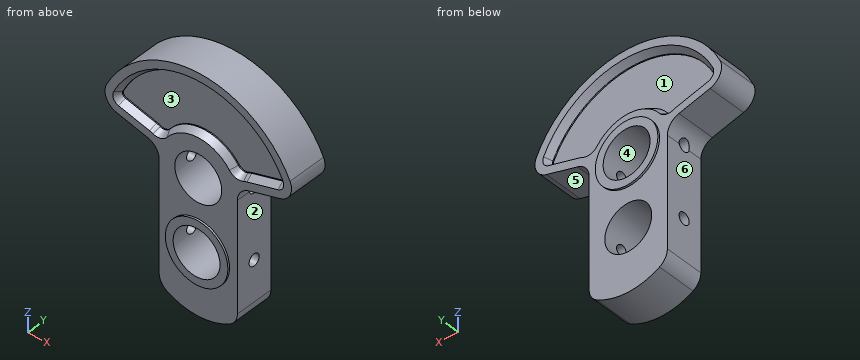
from build123d import *

# Parameters (mm, degrees)
BOSS_EXTRUDE1_DEPTH       = 5
FILLET1_R                 = 4
SKETCH2_R                 = 8
BOSS_EXTRUDE2_DEPTH       = 0.5
SKETCH3_R                 = 8
BOSS_EXTRUDE3_DEPTH       = 0.5
SKETCH4_R                 = 6
CUT_EXTRUDE1_DEPTH        = 43.969085178
CUT_EXTRUDE2_DEPTH        = 2
FILLET3_R                 = 2
CHAMFER1_SIZE             = 1
CHAMFER1_SIZE2            = 1.732050808
FILLET3_OF_MIRROR9_R      = 2
CHAMFER1_OF_MIRROR9_SIZE2 = 1.732050808
CHAMFER1_OF_MIRROR9_SIZE  = 1
CUT_EXTRUDE3_DEPTH        = 42.899788694
CUT_EXTRUDE3_DEPTH_BACK   = 42.899788694
SKETCH7_R                 = 1.5


with BuildPart() as part:
    # Sketch1 → Boss-Extrude1 (new, symmetric)
    with BuildSketch(Plane(origin=(0, 0, 0), x_dir=(1, 0, 0), z_dir=(0, 1, 0))):
        with BuildLine():
            Line((10, 0), (10, 30.489995997))
            ThreePointArc((10, 30.489995997), (0, 34), (-10, 30.489995997))
            Line((-10, 30.489995997), (-10, 0))
            Line((-10, 0), (-10, -2.679491924))
            Line((-10, -2.679491924), (-25.114071484, -6.729295173))
            ThreePointArc((-25.114071484, -6.729295173), (0, -26), (25.114071484, -6.729295173))
            Line((25.114071484, -6.729295173), (10, -2.679491924))
            Line((10, -2.679491924), (10, 0))
        make_face()
    extrude(amount=BOSS_EXTRUDE1_DEPTH, both=True)

    # Fillet1
    fillet1_edges = [part.edges().sort_by_distance(p)[0] for p in [
        (10, 0, 2.679491924),
        (25.114071484, 0, 6.729295173),
        (-25.114071484, 0, 6.729295173),
        (-10, 0, 2.679491924),
        (-10, 0, -30.489995997),
        (10, 0, -30.489995997),
    ]]
    fillet(fillet1_edges, radius=FILLET1_R)

    # Sketch2 → Boss-Extrude2 (add, symmetric)
    with BuildSketch(Plane(origin=(0, 5, 0), x_dir=(1, 0, 0), z_dir=(0, 1, 0))):
        with Locations(Location((0, 0, 0), (0, 0, 90))):
            Circle(SKETCH2_R)
    extrude(amount=BOSS_EXTRUDE2_DEPTH, both=True)

    # Sketch3 → Boss-Extrude3 (add, symmetric)
    with BuildSketch(Plane.XZ.offset(5)):
        with Locations(Location((0, -18, 0), (0, 0, 270))):
            Circle(SKETCH3_R)
    extrude(amount=BOSS_EXTRUDE3_DEPTH, both=True)

    # Sketch4 → Cut-Extrude1 (cut, through all)
    with BuildSketch(Plane(origin=(0, 5.5, 0), x_dir=(1, 0, 0), z_dir=(0, 1, 0))):
        with Locations(Location((0, 0, 0), (0, 0, 270))):
            Circle(SKETCH4_R)
        with Locations(Location((0, 18, 0), (0, 0, 270))):
            Circle(SKETCH4_R)
    extrude(amount=-CUT_EXTRUDE1_DEPTH, mode=Mode.SUBTRACT)

    # Sketch5 → Cut-Extrude2 (cut)
    with BuildSketch(Plane.XZ.offset(5)):
        with BuildLine():
            ThreePointArc((-9.720237296, 5.14946472), (-10.893551196, 5.883139881), (-12.188266684, 6.371664756))
            Line((-12.188266684, 6.371664756), (-20.119713435, 8.496889508))
            ThreePointArc((-20.119713435, 8.496889508), (-20.768948696, 9.043962883), (-20.763662316, 9.892943304))
            ThreePointArc((-20.763662316, 9.892943304), (0, 23), (20.763662316, 9.892943304))
            ThreePointArc((20.763662316, 9.892943304), (20.768948696, 9.043962883), (20.119713435, 8.496889508))
            Line((20.119713435, 8.496889508), (12.188266684, 6.371664756))
            ThreePointArc((12.188266684, 6.371664756), (10.893551196, 5.883139881), (9.720237296, 5.14946472))
            ThreePointArc((9.720237296, 5.14946472), (0, 11), (-9.720237296, 5.14946472))
        make_face()
    cut_extrude2 = extrude(amount=-CUT_EXTRUDE2_DEPTH, mode=Mode.SUBTRACT)

    # Fillet3
    fillet3_edges = [part.edges().sort_by_distance(p)[0] for p in [
        (-9.720237296, -4, 5.14946472),
        (9.720237296, -4, 5.14946472),
    ]]
    fillet(fillet3_edges, radius=FILLET3_R)

    # Chamfer1
    chamfer1_edges = [part.edges().sort_by_distance(p)[0] for p in [
        (0, -5, 11),
        (-11.674313174, -5, 6.212545731),
        (-9.864646178, -5, 5.908245307),
        (9.864646178, -5, 5.908245307),
        (-16.153990059, -5, 7.434277132),
        (16.153990059, -5, 7.434277132),
        (11.674313174, -5, 6.212545731),
        (20.768948696, -5, 9.043962883),
        (0, -5, 23),
        (-20.768948696, -5, 9.043962883),
    ]]
    chamfer1_side = [part.faces().sort_by_distance(p)[0] for p in [
        (-11.929022401, -5, 5.489455054),
    ]]
    chamfer(chamfer1_edges, length=CHAMFER1_SIZE, length2=CHAMFER1_SIZE2, reference=chamfer1_side[0])

    # Mirror9: Cut-Extrude2 across plane
    add(cut_extrude2.mirror(Plane.ZX), mode=Mode.SUBTRACT)

    # Fillet3 of Mirror9
    fillet3_of_mirror9_edges = [part.edges().sort_by_distance(p)[0] for p in [
        (-9.720237296, 4, 5.14946472),
        (9.720237296, 4, 5.14946472),
    ]]
    fillet(fillet3_of_mirror9_edges, radius=FILLET3_OF_MIRROR9_R)

    # Chamfer1 of Mirror9
    chamfer1_of_mirror9_edges = [part.edges().sort_by_distance(p)[0] for p in [
        (0, 5, 11),
        (-11.674313174, 5, 6.212545731),
        (-9.864646178, 5, 5.908245307),
        (9.864646178, 5, 5.908245307),
        (-16.153990059, 5, 7.434277132),
        (16.153990059, 5, 7.434277132),
        (11.674313174, 5, 6.212545731),
        (20.768948696, 5, 9.043962883),
        (0, 5, 23),
        (-20.768948696, 5, 9.043962883),
    ]]
    chamfer(chamfer1_of_mirror9_edges, length=CHAMFER1_OF_MIRROR9_SIZE, length2=CHAMFER1_OF_MIRROR9_SIZE2)

    # Sketch7 → Cut-Extrude3 (cut, two sides: drawn at the far end of the back side and taken through both)
    with BuildSketch(Plane(origin=(0, 0, 0), x_dir=(0, 0, -1), z_dir=(1, 0, 0)).offset(-CUT_EXTRUDE3_DEPTH_BACK)):
        with Locations((18, 0)):
            Circle(SKETCH7_R)
        Circle(SKETCH7_R)
    extrude(amount=CUT_EXTRUDE3_DEPTH + CUT_EXTRUDE3_DEPTH_BACK, mode=Mode.SUBTRACT)


solid = part.part
The listing builds one solid part. Answer for the finished solid, in the listing's coordinates (mm). Face numbers are marked on the shaded views. A direction names the side the tool comes from. Coordinates: 2 decimals unless noted, no trailing zeros. Write each loop counter-clockwise with the first axis right and the second up, starting at its lowest first coordinate (ties: lowest second). Pieces come first, ordered by that corner, then holes. Notation, with made-up numbers: (73, 22) - (121, 22) arc R18 cw to (121, 38) - close; hole circle Ø8 at (11, 89.5). An arc over 180 degrees is marked (long way). Return JSON: item names as keys, results as strings.
1. Which of the six approach directions +Z, -Z, +X, -X, +Y, -Y give full straight-line access (tool end or side, diameter ignored) to the marked faces 1, 2 and 3?
Final values:
{"face 1": "+Y", "face 2": "-Z, +X, +Y, -Y", "face 3": "-Y"}
2. For a pull along Z with two mould halves and no side action, classify the marked faces 4, 5 and 6 as +Z half, -Z half, draft (parallel to the pull), parting line (faces both ways), or undercut.
Final values:
{"face 4": "undercut", "face 5": "-Z half", "face 6": "draft"}
3. The part is cut by section C-C on x = 0. Count the separate pieces of the cut face and the enclosed holes in it, then the cut area to 3 significant figures.
Final values:
{"separate pieces": "3", "enclosed holes": "0", "area": "313 mm^2"}
4. Each of these flat-tipped pins is pushed along its axis until it touches: pin 1 Ø5 at (y, z) = (-1, -21) entering from +X; pin 2 Ø1.8 at (y, z) = (0, -18) entering from -X; pin 3 Ø19 at (x, z) = (5.5, 15) entering from -Y; pin 4 Ø5 at (x, z) = (8, 15.5) entering from +Y. Where does it stop, or does it pass through?
Final values:
{"pin 1": "x = 10", "pin 2": "through", "pin 3": "y = -5", "pin 4": "y = 3"}
5. The part is cut by section A-A on y = 0. Determine the outline of the cut face in (x, z).
Final values:
{"outline": "(-23.47, 11.18) arc R4 ccw to (-20.9, 5.6) - (-12.96, 3.47) arc R4 cw to (-10.47, 1.5) - (-5.81, 1.5) arc R6 cw to (5.81, 1.5) - (10.47, 1.5) arc R4 cw to (12.96, 3.47) - (20.9, 5.6) arc R4 ccw to (23.47, 11.18) arc R26 ccw to start; (-10, -28.39) arc R4 ccw to (-8, -31.86) arc R16 ccw to (8, -31.86) arc R4 ccw to (10, -28.39) - (10, -19.5) - (5.81, -19.5) arc R6 cw to (-5.81, -19.5) - (-10, -19.5) - close; (-10, -16.5) - (-5.81, -16.5) arc R6 cw to (5.81, -16.5) - (10, -16.5) - (10, -1.5) - (5.81, -1.5) arc R6 cw to (-5.81, -1.5) - (-10, -1.5) - close"}
6. Consider line 1 along X through (y, z) = (1.75, -16.5); line 2 along Z through (x, y) = (9, 0); line 3 along Z through (x, y) = (-8.75, 0). Determine where each line is inside the solid, lowest interval first.
Final values:
{"line 1": "-10 to -5.81, 5.81 to 10", "line 2": "-31.04 to -19.5, -16.5 to -1.5, 1.5 to 24.39", "line 3": "-31.3 to -19.5, -16.5 to -1.5, 1.5 to 24.48"}
7. The part is cut by section B-B on z = -18. Determine the outline of the cut face in (x, y).
Final values:
{"outline": "(-10, -5) - (-8, -5) - (-8, -5.5) - (-6, -5.5) - (-6, -1.5) - (-10, -1.5) - close; (-10, 1.5) - (-6, 1.5) - (-6, 5) - (-10, 5) - close; (6, -5.5) - (8, -5.5) - (8, -5) - (10, -5) - (10, -1.5) - (6, -1.5) - close; (6, 1.5) - (10, 1.5) - (10, 5) - (6, 5) - close"}
